Verification items for the finished model (mm, model axes). Give positions to 0.01 mm unless a question says otherwise; leave off trailing zeros. Loops run counter-clockwise (first coordinate to the right, second up) from the corner with the lowest first, then second, coordinate; pieces in that order, holes last. Notation, with made-up numbers: M -33.5,-38 L -16.5,-38 A9 cw -16.5,-28 Z; hole C 89,-15.5 d2. An arc over 180 degrees is marked long. Use a Markdown table: item, result.
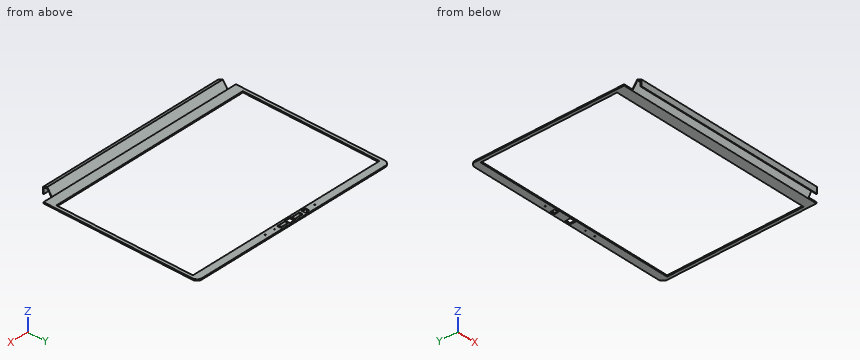
from build123d import *

# Parameters (mm, degrees)
SKETCH009_R   = 0.625
SKETCH009_R_2 = 0.75
SKETCH009_W   = 287.63
SKETCH009_H   = 192.5
SKETCH009_W_2 = 8
SKETCH009_H_2 = 8
SKETCH009_W_3 = 6
SKETCH009_H_3 = 6
PAD002_DEPTH  = 1.78
SKETCH_W      = 12.25
SKETCH_H      = 4.75
SKETCH_W_2    = 10
SKETCH_H_2    = 4.25
POCKET_DEPTH  = 1.7799
PAD_START     = 12.9
PAD_DEPTH     = 270.83


with BuildPart() as part:
    # Sketch009 → Pad002 (new body)
    with BuildSketch(Plane.XY.offset(12.53)):
        with BuildLine():
            Line((7, 228.98), (289.63, 228.98))
            ThreePointArc((296.63, 221.98), (294.579747, 226.929747), (289.63, 228.98))
            Line((296.63, 221.98), (296.63, 11.98))
            Line((296.63, 11.98), (0, 11.98))
            Line((0, 11.98), (0, 221.98))
            ThreePointArc((7, 228.98), (2.050253, 226.929747), (0, 221.98))
        make_face()
        with Locations((171.565, 223.48)):
            Circle(SKETCH009_R, mode=Mode.SUBTRACT)
        with Locations((185.815, 223.48)):
            Circle(SKETCH009_R_2, mode=Mode.SUBTRACT)
        with Locations((109.815, 223.48)):
            Circle(SKETCH009_R_2, mode=Mode.SUBTRACT)
        with Locations((148.315, 122.23)):
            Rectangle(SKETCH009_W, SKETCH009_H, mode=Mode.SUBTRACT)
        with Locations((148.315, 223.48)):
            Rectangle(SKETCH009_W_2, SKETCH009_H_2, mode=Mode.SUBTRACT)
        with Locations((124.315, 223.48)):
            Rectangle(SKETCH009_W_3, SKETCH009_H_3, mode=Mode.SUBTRACT)
    extrude(amount=-PAD002_DEPTH)

    # Sketch (on Sketch) → Pocket (cut)
    with BuildSketch(Plane.XY.offset(12.53)):
        with Locations((137.19, 223.855)):
            Rectangle(SKETCH_W, SKETCH_H)
        with Locations((138.065, 223.855)):
            Rectangle(SKETCH_W_2, SKETCH_H_2, mode=Mode.SUBTRACT)
        with Locations((159.44, 223.855)):
            Rectangle(SKETCH_W, SKETCH_H)
        with Locations((158.565, 223.855)):
            Rectangle(SKETCH_W_2, SKETCH_H_2, mode=Mode.SUBTRACT)
    extrude(amount=-POCKET_DEPTH, mode=Mode.SUBTRACT)

    # Sketch010 → Pad (join)
    with BuildSketch(Plane.YZ.offset(PAD_START)):
        Polygon((11.98, 12.53), (5.383871, 21.950249), (-0.621346, 19.462806), (-0.621346, 10.75), (0.378654, 10.75), (0.378654, 18.794628), (5.025063, 20.719233), (11.98, 10.75), align=None)
    extrude(amount=PAD_DEPTH)


solid = part.part
(1) Cross-section at C-C on z = 15. Record the cut outline in (x, y).
Results below:
| item | result |
|---|---|
| outline | M 12.9,-0.62 L 283.73,-0.62 L 283.73,0.38 L 12.9,0.38 Z; M 12.9,9.02 L 283.73,9.02 L 283.73,10.25 L 12.9,10.25 Z |
(2) Gauge pin test, flat ends, axial feed: P1, Ø5.5, axis at y = 8.5, z = 14.5, coming from the -X side; P2, Ø5, axis at x = 223.5, z = 20.5, coming from the +Y side; P3, Ø4.5, axis at x = 138, y = 224, coming from the +Z side; P4, Ø6, axis at y = 37.5, z = 13, coming from the +X side. Record the tip position at first contact, or that the pin passes through.
Results below:
| item | result |
|---|---|
| P1 | x = 12.9 |
| P2 | y = 8.15 |
| P3 | z = 12.53 |
| P4 | x = 296.63 |
(3) Cross-section at A-A on y = 199.5. Record the cut outline in (x, z).
Results below:
| item | result |
|---|---|
| outline | M 0,10.75 L 4.5,10.75 L 4.5,12.53 L 0,12.53 Z; M 292.13,10.75 L 296.63,10.75 L 296.63,12.53 L 292.13,12.53 Z |
(4) Material ranges on line 1 (X direction, y = 161, z = 11.5); line 2 (Y direction, x = 283, z = 12); line 3 (Y direction, x = 248.5, z = 18), recorded low to high.
Results below:
| item | result |
|---|---|
| line 1 | 0 to 4.5, 292.13 to 296.63 |
| line 2 | -0.62 to 0.38, 11.11 to 25.98, 218.48 to 228.98 |
| line 3 | -0.62 to 0.38, 6.92 to 8.15 |
(5) Cross-section at B-B on x = 180. Record the cut outline in (y, z), then the cut area to 3 significant figures.
Results below:
| item | result |
|---|---|
| outline | M -0.62,10.75 L 0.38,10.75 L 0.38,18.79 L 5.03,20.72 L 11.98,10.75 L 25.98,10.75 L 25.98,12.53 L 11.98,12.53 L 5.38,21.95 L -0.62,19.46 Z; M 218.48,10.75 L 228.98,10.75 L 228.98,12.53 L 218.48,12.53 Z |
| area | 69.7 mm^2 |
